Here's how the part is built. I have some questions about the finished solid (model axes, mm). A direction names the side the tool comes from. Round coordinates to 2 decimals unless told otherwise and drop trailing zeros. Write each loop counter-clockwise with the first axis right and the second up, starting at its lowest first coordinate (ties: lowest second). Pieces come first, ordered by that corner, then holes. Notation, with made-up numbers: M 42.5,8.5 L 92.5,8.5 A37 cw 92.5,46.5 Z; hole C -3.5,21.5 d8. An arc over 180 degrees is marked long. Use a Markdown table: item, result. Add a question column.
```python
from build123d import *

# Parameters (mm, degrees)
ESTRUSIONE_ESTRUSIONE1_DEPTH = 20
SCHIZZO2_R                   = 7.5
TAGLIO_ESTRUSIONE1_DEPTH     = 46.97825573
FORO_FILETTATO_M4_1_D        = 3.3
FORO_FILETTATO_M4_1_DEPTH    = 10.1
FORO_FILETTATO_M4_1_TIP      = 0.991420021


with BuildPart() as part:
    # Schizzo1 → Estrusione-Estrusione1 (new body)
    with BuildSketch(Plane.XY):
        Polygon((0, 0), (33, 0), (33, 12.5), (28, 12.5), (22, 18.5), (22, 25), (0, 25), align=None)
    extrude(amount=-ESTRUSIONE_ESTRUSIONE1_DEPTH)

    # Schizzo2 → Taglio-Estrusione1 (cut, through all)
    with BuildSketch(Plane.XZ):
        with Locations(Location((10.4, -10, 0), (0, 0, 270))):
            Circle(SCHIZZO2_R)
    extrude(amount=-TAGLIO_ESTRUSIONE1_DEPTH, mode=Mode.SUBTRACT)

    # Foro filettato M4-1
    with Locations(Plane(origin=(33, 0, 0), x_dir=(0, 0, -1), z_dir=(1, 0, 0))):
        with Locations((10, 6)):
            Hole(FORO_FILETTATO_M4_1_D / 2, depth=FORO_FILETTATO_M4_1_DEPTH)
            with Locations((0, 0, -(FORO_FILETTATO_M4_1_DEPTH + FORO_FILETTATO_M4_1_TIP / 2))):  # 118° drill point
                Cone(0, FORO_FILETTATO_M4_1_D / 2, FORO_FILETTATO_M4_1_TIP, mode=Mode.SUBTRACT)


solid = part.part
```
Item 1: Imagine slicing it at C-C on y = 17.25. List the corners of the cut face in (x, z) for me, plus the area to 3 significant figures.
Item 2: For pin 1 Ø3 at (y, z) = (6, -10) entering from +X; pin 2 Ø5 at (y, z) = (23, -7.5) entering from +X; pin 3 Ø4 at (x, z) = (31.5, -11.5) entering from +Y, each with a flat end and sliding along its axis, tell me the tip position at first contact or that it passes through.
Item 3: On a 3-axis mill with a long thin cutter (end or side, diameter ignored), from which of +Z, -Z, +X, -X, +Y, -Y can I reach the whole of each face in a straight line? I mean faces 1 (the face through (31, 12.5, -10)), 2 (the face through (20, 0, -10)). Say none if no direction works.
Item 4: Imagine slicing it at B-B on z = -14.5. List the corners of the cut face in (x, y) for me, plus the area to 4 significant figures.
Item 5: If we mould it in two halves opening along Y, with no side actions, what happens to faces 3 (the face through (27.879, 4.536, -9.239)), 4 (the face through (0, 13, -10)), 5 (the face through (14, 25, -3))? For each: +Y half, -Y half, draft (parallel to the pull), parting line (faces both ways), or undercut.
Item 6: I need wall thicknesses on probe 1 along X at (y, z) = (19.25, -10.25); probe 2 along Y at (x, z) = (31.25, -10); probe 3 along X at (y, z) = (11.25, -10). Which ranges of each line are inside material? Lowest first, please. Write a range as from..to.
Item 7: Imagine slicing it at A-A on x = 10.4. List the corners of the cut face in (y, z) for me.
Item 8: Imagine slicing it at D-D on z = -3. List the corners of the cut face in (x, y) for me, plus the area to 3 significant figures.
The answers:
| question | item | result |
|---|---|---|
| 1 | outline | M 0,-20 L 23.25,-20 L 23.25,0 L 0,0 Z; hole C 10.4,-10 d15 |
| 1 | area | 288 mm² |
| 2 | pin 1 | x = 22.81 |
| 2 | pin 2 | x = 22 |
| 2 | pin 3 | y = 12.5 |
| 3 | face 1 | +Z, -Z, +X, +Y |
| 3 | face 2 | +Z, -Z, +X, -X, -Y |
| 4 | outline | M 0,0 L 4.4,0 L 4.4,25 L 0,25 Z; M 16.4,0 L 33,0 L 33,12.5 L 28,12.5 L 22,18.5 L 22,25 L 16.4,25 Z |
| 4 | area | 405.5 mm² |
| 5 | face 3 | undercut |
| 5 | face 4 | draft |
| 5 | face 5 | +Y half |
| 6 | probe 1 | 0..2.9, 17.9..22 |
| 6 | probe 2 | 0..4.35, 7.65..12.5 |
| 6 | probe 3 | 0..2.9, 17.9..33 |
| 7 | outline | M 0,-20 L 25,-20 L 25,-17.5 L 0,-17.5 Z; M 0,-2.5 L 25,-2.5 L 25,0 L 0,0 Z |
| 8 | outline | M 0,0 L 7.71,0 L 7.71,25 L 0,25 Z; M 13.09,0 L 33,0 L 33,12.5 L 28,12.5 L 22,18.5 L 22,25 L 13.09,25 Z |
| 8 | area | 571 mm² |
